```python
from build123d import *

# Parameters (mm, degrees)
F0_W     = 350
F0_H     = 500
F1_DEPTH = 2
F2_SIZE  = 0.99999


# Not quite as in the source:
# - a fillet or chamfer is up to 0.001 mm smaller than in the source, because OpenCascade refuses the exact size


with BuildPart() as f1:
    # F0 (on Top) → F1 (new body)
    with BuildSketch(Plane.XY):
        Rectangle(F0_W, F0_H)
        Polygon((150, 100), (150, -100), (0, -100), (-150, -100), (-150, 100), (0, 100), align=None, mode=Mode.SUBTRACT)
        Polygon((-150, -100), (0, -100), (-150, 100), align=None)
        Polygon((0, 100), (150, -100), (150, 100), align=None)
        Polygon((-25, 0), (0, 100), (-150, 100), align=None)
        Polygon((0, -100), (150, -100), (25, 0), align=None)
    extrude(amount=F1_DEPTH)

    # F2 (size 1 in the source; OpenCascade refuses exactly that, so slightly less here)
    f2_edges = [f1.edges().sort_by_distance(p)[0] for p in [
        (-75, 0, 2),
        (-87.5, 50, 2),
        (-12.5, 50, 2),
        (75, 0, 2),
        (87.5, -50, 2),
        (12.5, -50, 2),
        (0, -250, 2),
        (175, 0, 2),
        (0, 250, 2),
        (-175, 0, 2),
        (-75, 0, 0),
        (-87.5, 50, 0),
        (-12.5, 50, 0),
        (75, 0, 0),
        (87.5, -50, 0),
        (12.5, -50, 0),
        (0, -250, 0),
        (175, 0, 0),
        (0, 250, 0),
        (-175, 0, 0),
        (-175, -250, 1),
        (175, -250, 1),
        (-175, 250, 1),
    ]]
    chamfer(f2_edges, length=F2_SIZE)


solid = f1.part
```
Part model, mm, in its own coordinate system. A direction names the side the tool comes from. Coordinates: 2 decimals unless noted, no trailing zeros. Order: outer loops, then holes, each group sorted by start corner. A loop starts at its lowest first (then second) coordinate and runs counter-clockwise, first axis right, second up. Notation, with made-up numbers: (43.5, 59) -> (61.5, 59) arc R9 cw to (61.5, 74) -> close; hole circle Ø1 at (69.25, 84). An arc over 180 degrees is marked (long way). Put each result on its own line as item: value. Start each with the question number.
(1) Probe line 1 along X through (y, z) = (-57.5, 1.25); line 2 along Y through (x, z) = (111.5, 1.75); line 3 along X through (y, z) = (28.5, 0.9). List the from-to ranges inside material, lowest first. Write a range as [from, to].
(2) Band-saw the part on C-C (z = 1.4). Give the cut face in (x, y), then the cut area to 3 significant figures.
(3) Mould opens along Y. For faces 1 (the face through (-41, 59, 0)), 2 (the face through (91.2, -53.6, 1.5)) say: pulls with the +Y half, pulls with the -Y half, needs draft (parallel to the pull), parting line crosses it, or undercut.
(4) Which spindle directions (+Z, -Z, +X, -X, +Y, -Y) get a long thin tool onto all of the face, cutting with end or side? Do faces 3 (the face through (-41, 59, 2)), 4 (the face through (-76.05, 0.55, 0.49)), 5 (the face through (12.92, -50.43, 1.51)). Say none if no direction does.
(5) Band-saw the part on A-A (y = -53). Count the separate pieces of the cut face and the enclosed holes in it, then the cut area to 3 significant figures.
Determined:
1. line 1: x = [-174.75, -32.19], [10.88, 96.47], [118.44, 174.75]
1. line 2: y = [-249.25, -70.16], [-47.42, 249.25]
1. line 3: x = [-174.9, -96.5], [-60.46, -17.98], [53.75, 174.9]
2. outline: (-174.6, -249) -> (-174, -249.6) -> (174, -249.6) -> (174.6, -249) -> (174.6, 249.6) -> (-174, 249.6) -> (-174.6, 249) -> close; hole (-152.21, 102.28) -> (0.18, -100.91) -> (25.24, -0.7) -> (152.21, -102.28) -> (-0.18, 100.91) -> (-25.24, 0.7) -> close
2. area: 159,000 mm²
3. face 1: needs draft
3. face 2: undercut
4. face 3: +Z, +X, -X, +Y, -Y
4. face 4: -Z
4. face 5: +Z
5. separate pieces: 3
5. enclosed holes: 0
5. area: 552 mm²
